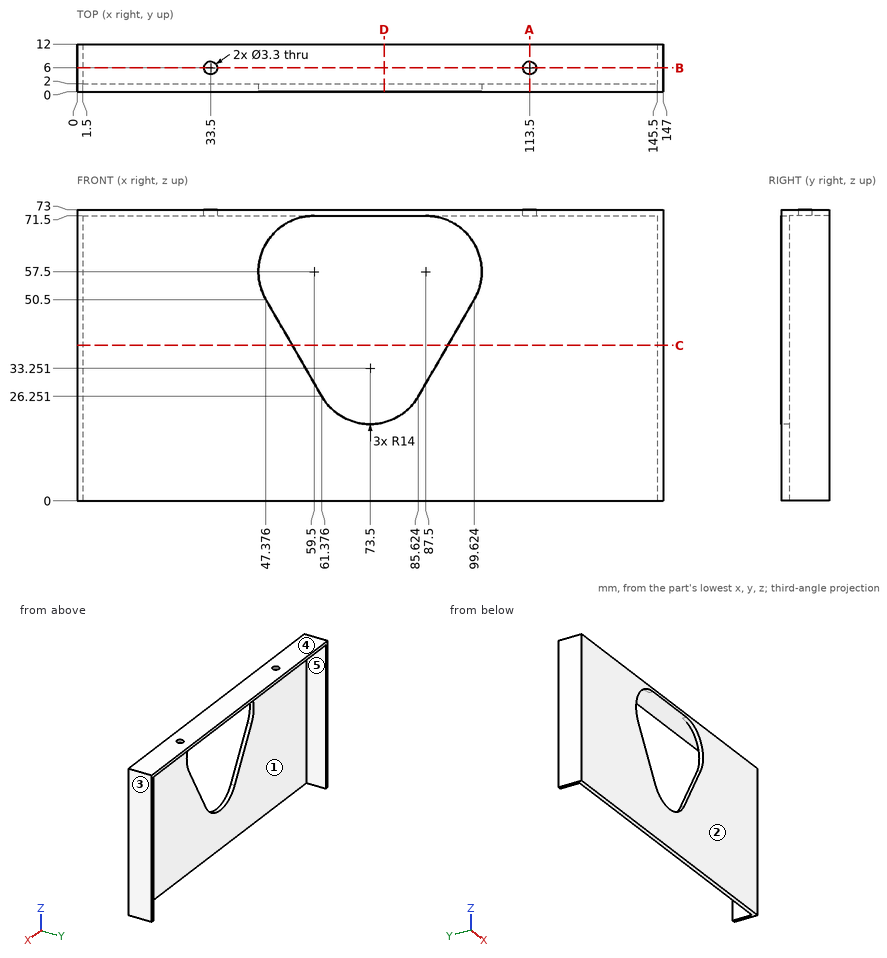
The figure shows three views and two pictorial views of one solid part (mm, origin at its lowest corner). Answer the questions. A direction names the side the tool comes from. Coordinates: 2 decimals unless noted, no trailing zeros. Loops run counter-clockwise (first coordinate to the right, second up) from the corner with the lowest first, then second, coordinate; pieces in that order, holes last. Notation, with made-up numbers: (67, 35.25) -> (71, 35.25) arc R21 cw to (71, 46.25) -> close; hole circle Ø7 at (34, 6.25). An arc over 180 degrees is marked (long way). Return JSON: item names as keys, results as strings. Group by question number.
(1) A cutting plane is placed at D-D on x = 77. Write down the section's boundary in (y, z).
(2) Which of the six approach directions +Z, -Z, +X, -X, +Y, -Y give full straight-line access (tool end or side, diameter ignored) to the marked faces 1 and 2?
(3) A cutting plane is placed at B-B on y = 6. Write down the section's boundary in (x, z).
(4) Given pin 1 Ø6 at (y, z) = (8.5, 31) entering from -X; pin 2 Ø5.5 at (x, y) = (33.5, 6) entering from -Z, each flat-ended and moving along its own axis, determine where each tip first touches the part or whether it passes through.
(5) Find the intervals of material crossed by probe 1 along X at (y, z) = (4.25, 29.5); probe 2 along Y at (x, z) = (33.5, 72.05); probe 3 along Z at (x, y) = (110.5, 9.25), in increasing order. Write a range as from..to.
(6) A cutting plane is placed at C-C on z = 39. Write down the section's boundary in (x, y) (1 decimal), and give its area (3 significant figures).
(7) Determine the mould class of the marked faces 3, 4 and 5 for opening direction X: released by +X, released by -X, zero draft, split by the parting line, or undercut.
(8) A cutting plane is placed at A-A on x = 113.5. Write down the section's boundary in (y, z).
The answers:
{
 "1": {"outline": "(0, 0) -> (2, 0) -> (2, 19.7) -> (0, 19.7) -> close; (0, 71.5) -> (12, 71.5) -> (12, 73) -> (0, 73) -> close"},
 "2": {"face 1": "-Z, +Y", "face 2": "+Z, -Z, +X, -X, -Y"},
 "3": {"outline": "(0, 0) -> (1.5, 0) -> (1.5, 71.5) -> (31.85, 71.5) -> (31.85, 73) -> (0, 73) -> close; (35.15, 71.5) -> (111.85, 71.5) -> (111.85, 73) -> (35.15, 73) -> close; (115.15, 71.5) -> (145.5, 71.5) -> (145.5, 0) -> (147, 0) -> (147, 73) -> (115.15, 73) -> close"},
 "4": {"pin 1": "stops at x = 0", "pin 2": "stops at z = 71.5"},
 "5": {"probe 1": "x = 0..1.5, 145.5..147", "probe 2": "y = 0..4.35, 7.65..12", "probe 3": "z = 71.5..73"},
 "6": {"outline": "(0, 0) -> (54, 0) -> (54, 2) -> (1.5, 2) -> (1.5, 12) -> (0, 12) -> close; (93, 0) -> (147, 0) -> (147, 12) -> (145.5, 12) -> (145.5, 2) -> (93, 2) -> close", "area": "246 mm^2"},
 "7": {"face 3": "released by +X", "face 4": "zero draft", "face 5": "undercut"},
 "8": {"outline": "(0, 0) -> (2, 0) -> (2, 71.5) -> (4.35, 71.5) -> (4.35, 73) -> (0, 73) -> close; (7.65, 71.5) -> (12, 71.5) -> (12, 73) -> (7.65, 73) -> close"}
}
